```python
from build123d import *

# Parameters (mm, degrees)
SKETCH_1_W          = 250
SKETCH_1_H          = 100
EXTRUDE_1_DEPTH     = 370
CUT_EXTRUDE_1_DEPTH = 370
CUT_EXTRUDE_3_DEPTH = 458.602447546
FILLET_1_R          = 10
SHELL_2_T           = -1.2


with BuildPart() as part:
    # 草圖1 → 填料-伸長1 (new body)
    with BuildSketch(Plane.XY):
        Rectangle(SKETCH_1_W, SKETCH_1_H)
    extrude(amount=EXTRUDE_1_DEPTH)

    # 草圖2 → 除料-伸長1 (cut)
    with BuildSketch(Plane.XY.offset(370)):
        Polygon((-125, 50), (-100, -50), (-125, -50), align=None)
        Polygon((125, 50), (125, -50), (100, -50), align=None)
    extrude(amount=-CUT_EXTRUDE_1_DEPTH, mode=Mode.SUBTRACT)

    # 草圖7 → 除料-伸長3 (cut, through all)
    with BuildSketch(Plane(origin=(-125, 50, 370), x_dir=(0, 0, 1), z_dir=(-1, 0, 0))):
        Polygon((0, 0), (-15, -100), (0, -100), align=None)
        Polygon((-370, 0), (-265, -100), (-370, -100), align=None)
    extrude(amount=-CUT_EXTRUDE_3_DEPTH, mode=Mode.SUBTRACT)

    # 圓角1
    fillet_1_edges = [part.edges().sort_by_distance(p)[0] for p in [
        (112.5, 0, 362.5),
        (0, -50, 355),
        (-112.5, 0, 362.5),
        (100, -50, 230),
        (112.5, 0, 52.5),
        (-100, -50, 230),
        (-112.5, 0, 52.5),
        (0, -50, 105),
    ]]
    fillet(fillet_1_edges, radius=FILLET_1_R)

    # 薄殼2
    shell_2_openings = [part.faces().sort_by_distance(p)[0] for p in [
        (0, 50, 185.000169968),
    ]]
    offset(amount=SHELL_2_T, openings=shell_2_openings, kind=Kind.INTERSECTION)


solid = part.part
```
Could you check a few things on this model? Use its own coordinates, in mm. A direction names the side the tool comes from. Coordinates: 2 decimals unless noted, no trailing zeros. Write each loop counter-clockwise with the first axis right and the second up, starting at its lowest first coordinate (ties: lowest second). Pieces come first, ordered by that corner, then holes. Notation, with made-up numbers: M -29,-4.5 L 10,-4.5 A4 cw 10,1.5 Z; hole C 17,53 d1. An arc over 180 degrees is marked long. Answer as CSV lines item,"result". Start each with the question number.
1) For P1, Ø8, axis at x = 33, y = -10, coming from the -Z side; P2, Ø10, axis at x = 32.5, y = 5.5, coming from the +Z side (3 decimals); P3, Ø5, axis at y = 28.5, z = 82, coming from the -X side, each with a flat end and sliding along its axis, tell me the tip position at first contact or that it passes through.
2) Please list where these lines run through material, in increasing order: line 1 (X direction, y = 27.5, z = 318) (3 decimals); line 2 (Z direction, x = -63, y = 37.5) (3 decimals); line 3 (X direction, y = 40.5, z = 108) (3 decimals). Write a range as from..to.
3) I want a section at A-A, the plane z = 271. Please give me the cut outline in (x, y).
4) For faces 1 (the cylindrical face through (-98.419, -47.825, 226.032)), 2 (the cylindrical face through (-109.719, 2.061, 55.133)), which set-ups out of +Z, -Z, +X, -X, +Y, -Y let a thin tool reach every point of the face, with its end or its side?
5) I want a section at B-B, the plane x = 27. Please give me the cut outline in (y, z), and give its area (3 significant figures).
6) We'd pull the mould along X, two halves only. Please class faces 3 (the flat face through (-113.6, 4.4, 227.2)), 4 (the cylindrical face through (110.056, 3.412, 53.714)), 5 (the flat face through (-1.631, 2.06, 50.337)), 6 (the cylindrical face through (-109.588, 3.2, 359.206)): +X half, -X half, draft (parallel to the pull), parting line (faces both ways), or undercut.
Data:
1,P1,"stops at z = 58.8"
1,P2,"stops at z = 364.075"
1,P3,"stops at x = -120.25"
2,line 1,"x = -119.375..-118.138, 118.138..119.375"
2,line 2,"z = 13.125..14.865, 366.912..368.125"
2,line 3,"x = -122.625..-121.388, 121.388..122.625"
3,outline,"M -125,50 L -101.89,-42.43 A10 ccw -92.19,-50 L 92.19,-50 A10 ccw 101.89,-42.43 L 125,50 L 123.76,50 L 100.73,-42.13 A8.8 cw 92.19,-48.8 L -92.19,-48.8 A8.8 cw -100.73,-42.13 L -123.76,50 Z"
4,face 1,"+Z, -Z, -X, -Y"
4,face 2,"+Y"
5,outline,"M -50,109 A10 ccw -47.24,102.1 L 50,0 L 50,1.74 L -46.37,102.93 A8.8 cw -48.8,109 L -48.8,346.39 A8.8 cw -41.31,355.09 L 50,368.79 L 50,370 L -41.48,356.28 A10 ccw -50,346.39 Z"
5,area,"589 mm^2"
6,face 3,"-X half"
6,face 4,"undercut"
6,face 5,"draft"
6,face 6,"undercut"
